from build123d import *

# Parameters (mm, degrees)
SKETCH1_R                   = 10.2489
BOSS_EXTRUDE1_DEPTH         = 2.9845
BOSS_EXTRUDE1_2_DEPTH       = 2.9845
SKETCH2_R                   = 10.2489
BOSS_EXTRUDE2_DEPTH         = 5.08
BOSS_EXTRUDE3_DEPTH         = 3.81
F_1_4_0_25_DIAMETER_HOLE1_D = 6.35
BOSS_EXTRUDE4_DEPTH         = 17.78
SKETCH8_R                   = 2.25
CUT_EXTRUDE1_DEPTH          = 17.78
SKETCH9_W                   = 17.78
SKETCH9_H                   = 2.54
BOSS_EXTRUDE5_DEPTH         = 17.78
CUT_EXTRUDE2_REACH          = 251.195
CUT_EXTRUDE3_DEPTH          = 20
BOSS_EXTRUDE6_DEPTH         = 2.54
BOSS_EXTRUDE7_DEPTH         = 39.624
F_6_CLEARANCE_HOLE1_D       = 3.7973
CUT_EXTRUDE4_DEPTH          = 6.35
SKETCH17_W                  = 39.624
SKETCH17_H                  = 20
BOSS_EXTRUDE8_DEPTH         = 6.35
M4_CLEARANCE_HOLE1_D        = 4.5
SKETCH21_R                  = 4.308
CUT_EXTRUDE5_DEPTH          = 195.822050963
FILLET2_R                   = 11
CUT_EXTRUDE6_DEPTH          = 6.35
BOSS_EXTRUDE9_DEPTH         = 21.844
CUT_EXTRUDE7_DEPTH          = 195.822050963


with BuildPart() as part:
    # Sketch1 → Boss-Extrude1 (new body)
    with BuildSketch(Plane.XY):
        Circle(SKETCH1_R)
    extrude(amount=BOSS_EXTRUDE1_DEPTH)



with BuildPart() as body_2:
    # Sketch1 → Boss-Extrude1 2 (new body)
    with BuildSketch(Plane.XY):
        with Locations((-72.411066703, 81.765798589)):
            Circle(SKETCH1_R)
    extrude(amount=BOSS_EXTRUDE1_2_DEPTH)


with BuildPart() as part_1:
    add(part.part)

    add(body_2.part)  # Boss-Extrude2 merges body 2
    # Sketch2 → Boss-Extrude2 (add)
    with BuildSketch(Plane.XY.offset(2.9845)):
        with Locations((-72.411066703, 81.765798589)):
            Circle(SKETCH2_R)
        Circle(SKETCH2_R)
    extrude(amount=BOSS_EXTRUDE2_DEPTH)

    # Sketch3 → Boss-Extrude3 (add)
    with BuildSketch(Plane.XY.offset(8.0645)):
        Polygon((-134.069705847, 103.500499391), (-96.039101852, 137.180065299), (52.150988145, -30.154592279), (14.12038415, -63.834158187), align=None)
    extrude(amount=BOSS_EXTRUDE3_DEPTH)

    # 1/4 (0.25) Diameter Hole1 (through all)
    with Locations(Plane.XY.offset(11.8745)):
        with Locations((0, 0), (-72.411066703, 81.765798589)):
            Hole(F_1_4_0_25_DIAMETER_HOLE1_D / 2)

    # Sketch7 → Boss-Extrude4 (add)
    with BuildSketch(Plane(origin=(0, 0, 8.0645), x_dir=(-1, 0, 0), z_dir=(0, 0, -1))):
        Polygon((66.604496657, 27.319509971), (61.850671158, 31.529455709), (48.59099954, 16.556776971), (53.34482504, 12.346831233), align=None)
        Polygon((-14.12038415, -63.834158187), (-0.860712533, -48.861479449), (-5.614538032, -44.65153371), (-18.87420965, -59.624212449), align=None)
    extrude(amount=BOSS_EXTRUDE4_DEPTH)

    # Sketch8 → Cut-Extrude1 (cut)
    with BuildSketch(Plane(origin=(-19.015301997, -16.839782954, 0), x_dir=(0, 0, -1), z_dir=(0.7486339369082557, 0.6629835808745536, 0))):
        with Locations(Location((4.6355, -47.15, 0), (0, 0, 90))):
            Circle(SKETCH8_R)
        with Locations(Location((0, 54.61, 0), (0, 0, 90))):
            Circle(SKETCH8_R)
    extrude(amount=-CUT_EXTRUDE1_DEPTH, mode=Mode.SUBTRACT)

    # Sketch9 → Boss-Extrude5 (add)
    with BuildSketch(Plane(origin=(-19.015301997, -16.839782954, 0), x_dir=(0, 0, -1), z_dir=(0.7486339369082557, 0.6629835808745536, 0))):
        with Locations((0.8255, -55.88)):
            Rectangle(SKETCH9_W, SKETCH9_H)
        with Locations((0.8255, 45.88)):
            Rectangle(SKETCH9_W, SKETCH9_H)
        with Locations((0.8255, 63.34)):
            Rectangle(SKETCH9_W, SKETCH9_H)
        with Locations((0.8255, -38.42)):
            Rectangle(SKETCH9_W, SKETCH9_H)
    extrude(amount=BOSS_EXTRUDE5_DEPTH)

    # Cut-Extrude2: up to this face of the body (flat: up to its plane)
    cut_extrude2_end = Plane(part_1.part.faces().sort_by_distance((9.892980981, -40.862582546, -0.8255))[0])
    # Sketch10 → Cut-Extrude2 (cut, up to the picked face)
    with BuildSketch(Plane(origin=(37.889511647, -42.784429494, 0), x_dir=(0.7486339369082557, 0.6629835808745536, 0), z_dir=(0.6629835808745536, -0.7486339369082557, 0)), mode=Mode.PRIVATE) as cut_extrude2_sk1:
        Polygon((-7.62, 8.0645), (-7.62, -9.7155), (-25.4, -9.7155), align=None)
    cut_extrude2_tool1 = split(extrude(cut_extrude2_sk1.sketch, amount=-CUT_EXTRUDE2_REACH, mode=Mode.PRIVATE), bisect_by=cut_extrude2_end, keep=Keep.BOTH, mode=Mode.PRIVATE)
    add(cut_extrude2_tool1.solids().sort_by(Axis((27.748017, -51.765647, -3.788833), (-0.6629835808745536, 0.7486339369082557, 0)))[0], mode=Mode.SUBTRACT)

    # Sketch11 → Cut-Extrude3 (cut)
    with BuildSketch(Plane(origin=(-29.575697543, 33.396559925, 0), x_dir=(0.748633936908256, 0.6629835808745533, 0), z_dir=(0.6629835808745533, -0.748633936908256, 0))):
        Polygon((-7.62, -9.7155), (-7.62, 8.0645), (-25.4, -9.7155), align=None)
    extrude(amount=-CUT_EXTRUDE3_DEPTH, mode=Mode.SUBTRACT)

    # Sketch12 → Boss-Extrude6 (add)
    with BuildSketch(Plane(origin=(37.889511647, -42.784429494, 0), x_dir=(0.7486339369082557, 0.6629835808745536, 0), z_dir=(0.6629835808745536, -0.7486339369082557, 0))):
        Polygon((-25.4, -9.7155), (19.05, -9.7155), (19.05, 8.0645), (-7.62, 8.0645), align=None)
    extrude(amount=-BOSS_EXTRUDE6_DEPTH)

    # Sketch13 → Boss-Extrude7 (add)
    with BuildSketch(Plane(origin=(0, 0, 8.0645), x_dir=(-1, 0, 0), z_dir=(0, 0, -1))):
        Polygon((96.039101852, 137.180065299), (134.069705847, 103.500499391), (125.64981437, 93.992848392), (87.619210375, 127.6724143), align=None)
    extrude(amount=BOSS_EXTRUDE7_DEPTH)

    # #6 Clearance Hole1 (through all)
    with Locations(Plane.XY.offset(11.8745)):
        with Locations((-120.35210911, 107.166565368), (-101.336807112, 124.006348323)):
            Hole(F_6_CLEARANCE_HOLE1_D / 2)

    # Sketch14 → Cut-Extrude4 (cut)
    with BuildSketch(Plane.XY.offset(11.8745)):
        Polygon((-106.55273324, 125.748757468), (-105.45374076, 120.360428364), (-97.219873465, 127.652268281), (-102.435799592, 129.394677426), align=None)
        Polygon((-97.219873465, 127.652268281), (-105.45374076, 120.360428364), (-100.237814632, 118.618019219), (-96.120880984, 122.263939177), align=None)
        Polygon((-125.568035237, 108.908974514), (-124.469042757, 103.52064541), (-116.235175462, 110.812485327), (-121.45110159, 112.554894472), align=None)
        Polygon((-116.235175462, 110.812485327), (-124.469042757, 103.52064541), (-119.25311663, 101.778236265), (-115.136182982, 105.424156223), align=None)
    extrude(amount=-CUT_EXTRUDE4_DEPTH, mode=Mode.SUBTRACT)

    # Sketch17 → Boss-Extrude8 (add)
    with BuildSketch(Plane(origin=(-23.769127497, -21.049728693, 0), x_dir=(0, 0, 1), z_dir=(-0.7486339369082559, -0.6629835808745536, 0))):
        with Locations((-11.7475, 150.02)):
            Rectangle(SKETCH17_W, SKETCH17_H)
    extrude(amount=-BOSS_EXTRUDE8_DEPTH)

    # M4 Clearance Hole1 (through all)
    with Locations(Plane(origin=(-19.015301997, -16.839782954, 0), x_dir=(0, 0, -1), z_dir=(0.7486339369082559, 0.6629835808745536, 0))):
        with Locations((1.8415, 150.02), (21.6535, 150.02)):
            Hole(M4_CLEARANCE_HOLE1_D / 2)

    # Sketch21 → Cut-Extrude5 (cut, through all)
    with BuildSketch(Plane(origin=(-19.015301997, -16.839782954, 0), x_dir=(0, 0, -1), z_dir=(0.7486339369082559, 0.6629835808745536, 0))):
        with Locations((21.6535, 150.02)):
            Circle(SKETCH21_R)
        with Locations((1.8415, 150.02)):
            Circle(SKETCH21_R)
    extrude(amount=CUT_EXTRUDE5_DEPTH, mode=Mode.SUBTRACT)

    # Fillet2
    # the kernel refuses this fillet: 11 mm, written as the material it adds along each edge
    with BuildSketch(Plane(origin=(50.46700985, -28.253062079, 8.0645), x_dir=(-0.6629835808745533, 0.7486339369082559, 1.2918958832001814e-15), z_dir=(-0.748633936908256, -0.6629835808745534, 0))) as fillet2_piece_1:
        with BuildLine():
            CenterArc((FILLET2_R, FILLET2_R), FILLET2_R, 180, 90)
            Line((0, FILLET2_R), (0, 0))
            Line((0, 0), (FILLET2_R, 0))
        make_face()
    extrude(amount=44.45)
    # the kernel refuses this fillet: 11 mm, written as the material it takes off along each edge
    with BuildSketch(Plane(origin=(72.73842141, -11.922543805, 11.8745), x_dir=(-0.6629835808745536, 0.7486339369082557, 0), z_dir=(-0.7486339369082559, -0.6629835808745537, 0))) as fillet2_2_piece_1:
        with BuildLine():
            CenterArc((FILLET2_R, FILLET2_R), FILLET2_R, 180, 90)
            Line((0, FILLET2_R), (0, 0))
            Line((0, 0), (FILLET2_R, 0))
        make_face()
    extrude(amount=105.8, mode=Mode.SUBTRACT)
    with BuildSketch(Plane(origin=(-154.657139112, 85.268450917, 11.8745), x_dir=(0, 0, -1), z_dir=(0.7486339369082557, 0.6629835808745537, 0))) as fillet2_2_piece_2:
        with BuildLine():
            CenterArc((FILLET2_R, -FILLET2_R), FILLET2_R, 90, 90)
            Line((0, -FILLET2_R), (0, 0))
            Line((0, 0), (FILLET2_R, 0))
        make_face()
    extrude(amount=105.8, mode=Mode.SUBTRACT)

    # Sketch22 → Cut-Extrude6 (cut)
    with BuildSketch(Plane.XY.offset(5.5245)):
        Polygon((-121.45110159, 112.554894472), (-125.568035237, 108.908974514), (-124.469042757, 103.52064541), (-119.25311663, 101.778236265), (-115.136182982, 105.424156223), (-116.235175462, 110.812485327), align=None)
        Polygon((-102.435799592, 129.394677426), (-106.55273324, 125.748757468), (-105.45374076, 120.360428364), (-100.237814632, 118.618019219), (-96.120880984, 122.263939177), (-97.219873465, 127.652268281), align=None)
    extrude(amount=-CUT_EXTRUDE6_DEPTH, mode=Mode.SUBTRACT)

    # Sketch24 → Boss-Extrude9 (add)
    with BuildSketch(Plane(origin=(0, 0, -9.7155), x_dir=(-1, 0, 0), z_dir=(0, 0, -1))):
        Polygon((-7.298516327, -46.55306391), (-17.190231354, -57.722682249), (-50.46700985, -28.253062079), (-52.150988145, -30.154592279), (-14.12038415, -63.834158187), (-0.860712533, -48.861479449), (-5.614538032, -44.65153371), align=None)
    extrude(amount=BOSS_EXTRUDE9_DEPTH)

    # Sketch25 → Cut-Extrude7 (cut, through all)
    with BuildSketch(Plane(origin=(-19.015301997, -16.839782954, 0), x_dir=(0, 0, -1), z_dir=(0.7486339369082557, 0.6629835808745536, 0))):
        with BuildLine():
            ThreePointArc((26.1535, -47.15), (25.494490258, -45.559009742), (23.9035, -44.9))
            Line((23.9035, -44.9), (23.9035, -47.15))
            Line((23.9035, -47.15), (21.6535, -47.15))
            ThreePointArc((21.6535, -47.15), (23.9035, -49.4), (26.1535, -47.15))
        make_face()
        with BuildLine():
            Line((23.9035, -47.15), (23.9035, -44.9))
            ThreePointArc((23.9035, -44.9), (22.312509742, -45.559009742), (21.6535, -47.15))
            Line((21.6535, -47.15), (23.9035, -47.15))
        make_face()
    extrude(amount=-CUT_EXTRUDE7_DEPTH, mode=Mode.SUBTRACT)


solid = part_1.part
For this review, take the finished solid that the model builds, in its own axes (mm). A direction names the side the tool comes from. Coordinates: 2 decimals unless noted, no trailing zeros. Order: outer loops, then holes, each group sorted by start corner. A loop starts at its lowest first (then second) coordinate and runs counter-clockwise, first axis right, second up. Notation, with made-up numbers: (-27, 54.25) - (11, 54.25) arc R11 ccw to (11, 66.25) - close; hole circle Ø10 at (73.25, 5.5). An arc over 180 degrees is marked (long way). Answer as CSV lines item,"result". Start each with the question number.
1) Add section A-A (y = 0). State the section outline as (x, z) points (1 decimal), then the cut area to 3 significant figures.
2) Insertion check: P1, Ø10, axis at x = 3.5, y = -4, coming from the -Z side; P2, Ø5, axis at x = -1.5, z = 1, coming from the -Y side; P3, Ø3, axis at x = -110.5, z = 0.5, coming from the +Y side; P4, Ø10, axis at x = -72.41, y = 81.77, coming from the +Z side. Each pin has a flat end and moves straight along its axis. Give the tip position at first contact, or say it passes through.
3) Add section C-C (y = 48). State the section outline as (x, z) points.
4) Add section B-B (x = -78). State the section outline as (y, z) points.
5) To check wall thickness, follow line 1 along Z through (x, y) = (17, -7.5); line 2 along X through (y, z) = (106.5, -6); line 3 along X through (y, z) = (-46, -15). State the ranges of each line that lie inside material, in increasing order. Write a range as [from, to].
6) Draft analysis for pull direction Y (two halves, no side actions). For faces 1 (the flat face through (25, -53, -31.56)), 2 (the flat face through (-54.248, 36.542, -0.701)), 3 (the flat face through (-115.678, 108.081, 5.613)), 4 (the flat face through (-96.663, 124.92, 5.613)), state which applies: +Y half, -Y half, draft (parallel to the pull), parting line (faces both ways), or undercut.
7) Machinability: for faces 5 (the flat face through (-121.898, 102.662, 5.613)), 6 (the flat face through (-104.49, 112.73, -11.64)), 7 (the cylindrical face through (-104.93, 113.22, -1.88)), 8 (the flat face through (-2.4, 2.4, 0)), which of the approach directions +Z, -Z, +X, -X, +Y, -Y give a long, thin tool a straight path to every point of the face, cutting with its end or side? Answer none if there is none.
Result:
1,outline,"(-42.4, 8.1) - (-10.2, 8.1) - (-10.2, 0) - (-3.2, 0) - (-3.2, 11.9) - (-42.4, 11.9) - close; (3.2, 0) - (10.2, 0) - (10.2, 8.1) - (25.4, 8.1) - (25.4, 11.9) - (3.2, 11.9) - close"
1,area,"348 mm^2"
2,P1,"z = 0"
2,P2,"y = -49.02"
2,P3,"y = 125.7"
2,P4,"z = 11.87"
3,outline,"(-84.92, 8.06) - (-17.06, 8.06) - (-17.06, 11.87) - (-84.92, 11.87) - close"
4,outline,"(40.19, 8.06) - (73.17, 8.06) - (73.17, 0) - (90.36, 0) - (90.36, 8.06) - (116.81, 8.06) - (116.81, 11.87) - (40.19, 11.87) - close"
5,line 1,"[8.06, 11.87]"
5,line 2,"[-130.68, -122.13], [-118.57, -111.53]"
5,line 3,"[4.09, 6.81], [30.43, 34.26]"
6,face 1,"draft"
6,face 2,"+Y half"
6,face 3,"undercut"
6,face 4,"undercut"
7,face 5,"+Z"
7,face 6,"-Z, +X"
7,face 7,"+X"
7,face 8,"-Z, +X, -X, +Y"
